from build123d import *

# Parameters (mm, degrees)
SKETCH1_W           = 148.2
SKETCH1_H           = 106.1
SKETCH1_R           = 1.6
SKETCH1_W_2         = 128.2
SKETCH1_H_2         = 86.1
BOSS_EXTRUDE1_DEPTH = 3
FILLET1_R           = 2
FILLET2_R           = 0.5
CUT_EXTRUDE3_REACH  = 93.182
SKETCH4_R           = 1.5


with BuildPart() as part:
    # Sketch1 → Boss-Extrude1 (new body)
    with BuildSketch(Plane(origin=(0, 0, 0), x_dir=(1, 0, 0), z_dir=(0, 1, 0))):
        Rectangle(SKETCH1_W, SKETCH1_H)
        with Locations(Location((-69.1, 48.05, 0), (0, 0, 270))):
            Circle(SKETCH1_R, mode=Mode.SUBTRACT)
        with Locations(Location((-69.1, -48.05, 0), (0, 0, 90))):
            Circle(SKETCH1_R, mode=Mode.SUBTRACT)
        with Locations(Location((69.1, 48.05, 0), (0, 0, 90))):
            Circle(SKETCH1_R, mode=Mode.SUBTRACT)
        with Locations(Location((69.1, -48.05, 0), (0, 0, 270))):
            Circle(SKETCH1_R, mode=Mode.SUBTRACT)
        Rectangle(SKETCH1_W_2, SKETCH1_H_2, mode=Mode.SUBTRACT)
    extrude(amount=BOSS_EXTRUDE1_DEPTH)

    # Fillet1
    fillet1_edges = [part.edges().sort_by_distance(p)[0] for p in [
        (-74.1, 1.5, -53.05),
        (74.1, 1.5, -53.05),
        (74.1, 1.5, 53.05),
        (-74.1, 1.5, 53.05),
    ]]
    fillet(fillet1_edges, radius=FILLET1_R)

    # Fillet2
    fillet2_edges = [part.edges().sort_by_distance(p)[0] for p in [
        (64.1, 1.5, 43.05),
        (64.1, 1.5, -43.05),
        (-64.1, 1.5, -43.05),
        (-64.1, 1.5, 43.05),
    ]]
    fillet(fillet2_edges, radius=FILLET2_R)

    # Sketch4 → Cut-Extrude3 (cut, up to next)
    with BuildSketch(Plane(origin=(0, 3, 0), x_dir=(-1, 0, 0), z_dir=(0, 1, 0)), mode=Mode.PRIVATE) as cut_extrude3_sk1:
        with Locations(Location((-32.3, -48.05, 0), (0, 0, 90))):
            Circle(SKETCH4_R)
    cut_extrude3_tool1 = extrude(cut_extrude3_sk1.sketch, amount=-CUT_EXTRUDE3_REACH, mode=Mode.PRIVATE) & part.part
    # Sketch4 → Cut-Extrude3 (cut, up to next)
    with BuildSketch(Plane(origin=(0, 3, 0), x_dir=(-1, 0, 0), z_dir=(0, 1, 0)), mode=Mode.PRIVATE) as cut_extrude3_sk2:
        with Locations(Location((44.1, -48.05, 0), (0, 0, 90))):
            Circle(SKETCH4_R)
    cut_extrude3_tool2 = extrude(cut_extrude3_sk2.sketch, amount=-CUT_EXTRUDE3_REACH, mode=Mode.PRIVATE) & part.part
    # Sketch4 → Cut-Extrude3 (cut, up to next)
    with BuildSketch(Plane(origin=(0, 3, 0), x_dir=(-1, 0, 0), z_dir=(0, 1, 0)), mode=Mode.PRIVATE) as cut_extrude3_sk3:
        with Locations(Location((44.1, 48.05, 0), (0, 0, 90))):
            Circle(SKETCH4_R)
    cut_extrude3_tool3 = extrude(cut_extrude3_sk3.sketch, amount=-CUT_EXTRUDE3_REACH, mode=Mode.PRIVATE) & part.part
    # Sketch4 → Cut-Extrude3 (cut, up to next)
    with BuildSketch(Plane(origin=(0, 3, 0), x_dir=(-1, 0, 0), z_dir=(0, 1, 0)), mode=Mode.PRIVATE) as cut_extrude3_sk4:
        with Locations(Location((-32.3, 48.05, 0), (0, 0, 90))):
            Circle(SKETCH4_R)
    cut_extrude3_tool4 = extrude(cut_extrude3_sk4.sketch, amount=-CUT_EXTRUDE3_REACH, mode=Mode.PRIVATE) & part.part
    add(cut_extrude3_tool1.solids().sort_by_distance((32.3, 3, -48.05))[0], mode=Mode.SUBTRACT)
    add(cut_extrude3_tool2.solids().sort_by_distance((-44.1, 3, -48.05))[0], mode=Mode.SUBTRACT)
    add(cut_extrude3_tool3.solids().sort_by_distance((-44.1, 3, 48.05))[0], mode=Mode.SUBTRACT)
    add(cut_extrude3_tool4.solids().sort_by_distance((32.3, 3, 48.05))[0], mode=Mode.SUBTRACT)


solid = part.part
Design review of the part built by this model. Coordinates are the model's own, in mm. A direction names the side the tool comes from. Round coordinates to 2 decimals unless told otherwise and drop trailing zeros. Write each loop counter-clockwise with the first axis right and the second up, starting at its lowest first coordinate (ties: lowest second). Pieces come first, ordered by that corner, then holes. Notation, with made-up numbers: (69.25, 73.5) - (96.25, 73.5) arc R28 cw to (96.25, 95.5) - close; hole circle Ø7 at (24.25, 74). An arc over 180 degrees is marked (long way). Return JSON: item names as keys, results as strings. Group by question number.
Item 1: We need section C-C on x = 32.3. Write out the cut boundary in (y, z).
Item 2: We need section B-B on z = -48.05. Write out the cut boundary in (x, y), and give its area (3 significant figures).
Item 3: The part is to be moulded in two halves that separate along Z. For faces 1 (the face through (-43.65, 1.52, 49.48)), 2 (the face through (-1, 1, 53.05)), 3 (the face through (-1, 1, -53.05)), 4 (the face through (74.1, 1, 1)), say which applies: pulls with the +Z half, pulls with the -Z half, needs draft (parallel to the pull), parting line crosses it, or undercut.
Item 4: We need section D-D on z = 37. Write out the cut boundary in (x, y), and give its area (3 significant figures).
Item 5: Insertion check: P1, Ø3.5, axis at x = -44.1, z = -48.05, coming from the -Y side. The pin has a flat end and moves straight along its axis. Give the tip position at first contact, or say it passes through.
Item 6: Machinability: for faces 5 (the face through (-1, 1, -43.05)), 6 (the face through (-1, 0, 46)), which of the approach directions +Z, -Z, +X, -X, +Y, -Y give a long, thin tool a straight path to every point of the face, cutting with its end or side? Answer none if there is none.
Item 7: For probe 1 along X at (y, z) = (1.1, -48.05); probe 2 along Z at (x, y) = (-69.1, 2.2); probe 3 along Z at (x, y) = (23, 2.65), list the stretches that pass through material, from the lowest coordinate up. Write a range as [from, to].
Item 8: We need section A-A on x = -52. Write out the cut boundary in (y, z), and give its area (3 significant figures).
Model answer:
{
 "1": {"outline": "(0, -53.05) - (3, -53.05) - (3, -49.55) - (0, -49.55) - close; (0, -46.55) - (3, -46.55) - (3, -43.05) - (0, -43.05) - close; (0, 43.05) - (3, 43.05) - (3, 46.55) - (0, 46.55) - close; (0, 49.55) - (3, 49.55) - (3, 53.05) - (0, 53.05) - close"},
 "2": {"outline": "(-74.1, 0) - (-70.7, 0) - (-70.7, 3) - (-74.1, 3) - close; (-67.5, 0) - (-45.6, 0) - (-45.6, 3) - (-67.5, 3) - close; (-42.6, 0) - (30.8, 0) - (30.8, 3) - (-42.6, 3) - close; (33.8, 0) - (67.5, 0) - (67.5, 3) - (33.8, 3) - close; (70.7, 0) - (74.1, 0) - (74.1, 3) - (70.7, 3) - close", "area": "407 mm²"},
 "3": {"face 1": "undercut", "face 2": "pulls with the +Z half", "face 3": "pulls with the -Z half", "face 4": "needs draft"},
 "4": {"outline": "(-74.1, 0) - (-64.1, 0) - (-64.1, 3) - (-74.1, 3) - close; (64.1, 0) - (74.1, 0) - (74.1, 3) - (64.1, 3) - close", "area": "60.0 mm²"},
 "5": {"P1": "stops at y = 0"},
 "6": {"face 5": "+Y, -Y", "face 6": "+Z, -Z, +X, -X, -Y"},
 "7": {"probe 1": "x = [-74.1, -70.7], [-67.5, -45.6], [-42.6, 30.8], [33.8, 67.5], [70.7, 74.1]", "probe 2": "z = [-53.05, -49.65], [-46.45, 46.45], [49.65, 53.05]", "probe 3": "z = [-53.05, -43.05], [43.05, 53.05]"},
 "8": {"outline": "(0, -53.05) - (3, -53.05) - (3, -43.05) - (0, -43.05) - close; (0, 43.05) - (3, 43.05) - (3, 53.05) - (0, 53.05) - close", "area": "60.0 mm²"}
}
